Input: part model. Units: mm. Frame: model coordinates. Round coordinates to 2 decimals unless told otherwise and drop trailing zeros. Order: outer loops, then holes, each group sorted by start corner. A loop starts at its lowest first (then second) coordinate and runs counter-clockwise, first axis right, second up. Notation, with made-up numbers: (-8.75, 26.5) -> (27.25, 26.5) arc R15 cw to (27.25, 37.5) -> close; hole circle Ø7 at (14.25, 67.5). An arc over 180 degrees is marked (long way). Use a Markdown table: item, result.
from build123d import *

# Parameters (mm, degrees)
SKETCH1_W           = 300
SKETCH1_H           = 200
BOSS_EXTRUDE1_DEPTH = 450
SHELL1_T            = 10
SKETCH2_R           = 22.84898586
SKETCH2_R_2         = 21.039403667
BOSS_EXTRUDE2_DEPTH = 30
SKETCH5_R           = 10.76282056
SKETCH5_R_2         = 14.175471805
BOSS_EXTRUDE3_DEPTH = 15
SKETCH6_R           = 21.039403667
BOSS_EXTRUDE4_DEPTH = 15


with BuildPart() as part:
    # Sketch1 → Boss-Extrude1 (new body)
    with BuildSketch(Plane.XY):
        Rectangle(SKETCH1_W, SKETCH1_H)
    extrude(amount=BOSS_EXTRUDE1_DEPTH)

    # Shell1 (no face opened: a closed hollow body)
    add(offset(amount=-SHELL1_T, mode=Mode.PRIVATE), mode=Mode.SUBTRACT)

    # Sketch2 → Boss-Extrude2 (add)
    # profile 1 of 2: a face of its own
    with BuildSketch(Plane.XY.offset(450)):
        with Locations((87.640110274, -29.828388409)):
            Circle(SKETCH2_R)
        with Locations((87.640110274, -29.828388409)):
            Circle(SKETCH2_R_2, mode=Mode.SUBTRACT)
    # profile 2 of 2: a face of its own
    with BuildSketch(Plane.XY.offset(450)):
        with BuildLine():
            Line((-19.065567849, 0), (-19.065567849, -29.828388409))
            ThreePointArc((-19.065567849, -29.828388409), (9.840293083, -58.734249341), (38.746154016, -29.828388409))
            Line((38.746154016, -29.828388409), (38.746154016, 0))
            ThreePointArc((38.746154016, 0), (9.840293083, 28.905860932), (-19.065567849, 0))
        make_face()
        with BuildLine():
            Line((-16.964069854, 0), (-16.964069854, -29.828388409))
            ThreePointArc((-16.964069854, -29.828388409), (9.840293083, -56.632751347), (36.644656021, -29.828388409))
            Line((36.644656021, -29.828388409), (36.644656021, 0))
            ThreePointArc((36.644656021, 0), (9.840293083, 26.804362938), (-16.964069854, 0))
        make_face(mode=Mode.SUBTRACT)
    extrude(amount=BOSS_EXTRUDE2_DEPTH)

    # Sketch5 → Boss-Extrude3 (add)
    with BuildSketch(Plane.XY.offset(450)):
        with BuildLine():
            Line((-16.964069854, 0), (-16.964069854, -29.828388409))
            ThreePointArc((-16.964069854, -29.828388409), (9.840293083, -56.632751347), (36.644656021, -29.828388409))
            Line((36.644656021, -29.828388409), (36.644656021, 0))
            ThreePointArc((36.644656021, 0), (9.840293083, 26.804362938), (-16.964069854, 0))
        make_face()
        with Locations((9.840293083, 0)):
            Circle(SKETCH5_R, mode=Mode.SUBTRACT)
        with Locations((9.840293083, -29.828388409)):
            Circle(SKETCH5_R_2, mode=Mode.SUBTRACT)
    extrude(amount=BOSS_EXTRUDE3_DEPTH)

    # Sketch6 → Boss-Extrude4 (add)
    with BuildSketch(Plane.XY.offset(450)):
        with Locations((87.640110274, -29.828388409)):
            Circle(SKETCH6_R)
    extrude(amount=BOSS_EXTRUDE4_DEPTH)


solid = part.part
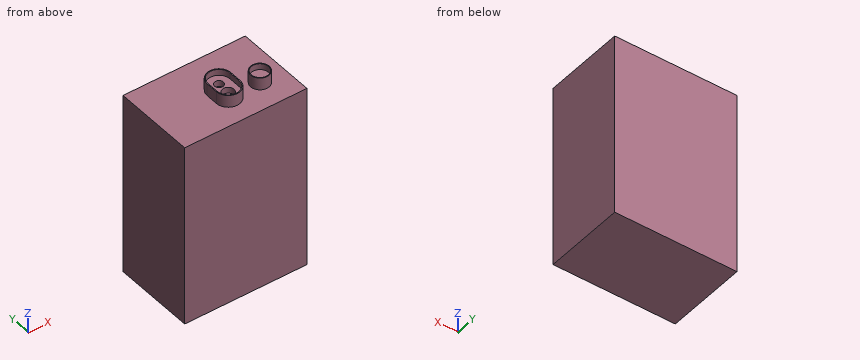
1) Cut plane B-B on x = -72.5. Return loops of the section in (y, z).
Results found:
| item | result |
|---|---|
| outline | (-100, 0) -> (100, 0) -> (100, 450) -> (-100, 450) -> close; hole (-90, 10) -> (90, 10) -> (90, 440) -> (-90, 440) -> close |
2) Pin query (flat end, axial travel): pin 1 Ø6 at (x, y) = (54, -42) entering from +Z; pin 2 Ø14 at (x, y) = (14, -36.5) entering from +Z; pin 3 Ø16.5 at (y, z) = (-16.5, 471.5) entering from +X. Return the tip coordinate at first contact, or that it passes through.
Results found:
| item | result |
|---|---|
| pin 1 | stops at z = 450 |
| pin 2 | stops at z = 465 |
| pin 3 | stops at x = 109.92 |
3) Cut plane A-A on z = 244. Return loops of the section in (x, y).
Results found:
| item | result |
|---|---|
| outline | (-150, -100) -> (150, -100) -> (150, 100) -> (-150, 100) -> close; hole (-140, -90) -> (140, -90) -> (140, 90) -> (-140, 90) -> close |
4) Line query: L1, parallel to Y at x = 70, z = 351; L2, parallel to Z at x = 64, y = -54.5; L3, parallel to X at y = -13.5, z = 111.5. Output: solid intervals per line, ascending. Write a range as [from, to].
Results found:
| item | result |
|---|---|
| L1 | y = [-100, -90], [90, 100] |
| L2 | z = [0, 10], [440, 450] |
| L3 | x = [-150, -140], [140, 150] |
5) Cut plane C-C on y = 19. Return loops of the section in (x, z), and give its area (3 significant figures).
Results found:
| item | result |
|---|---|
| outline | (-150, 0) -> (150, 0) -> (150, 450) -> (31.62, 450) -> (31.62, 480) -> (28.75, 480) -> (28.75, 465) -> (-9.07, 465) -> (-9.07, 480) -> (-11.94, 480) -> (-11.94, 450) -> (-150, 450) -> close; hole (-140, 10) -> (140, 10) -> (140, 440) -> (-140, 440) -> close |
| area | 15,300 mm² |
